Geometry check sheet. Reference: the model listing, model coordinates, mm. A direction names the side the tool comes from. Round coordinates to 2 decimals unless told otherwise and drop trailing zeros. Loops run counter-clockwise (first coordinate to the right, second up) from the corner with the lowest first, then second, coordinate; pieces in that order, holes last. Notation, with made-up numbers: M -25,86.25 L -9,86.25 A16 cw -9,98.25 Z; hole C 50.5,-26 d3. An arc over 180 degrees is marked long. Write item = value, one per line.
from build123d import *

# Parameters (mm, degrees)
SKETCH2_W            = 63.5
SKETCH2_H            = 63.5
BOSS_EXTRUDE1_DEPTH  = 2.54
BOSS_EXTRUDE2_DEPTH  = 2.54
SKETCH4_R            = 1.27
CUT_EXTRUDE1_DEPTH   = 2.54
BOSS_EXTRUDE3_DEPTH  = 2.54
BOSS_EXTRUDE4_DEPTH  = 2.54
EXTRUDE_THIN1_DEPTH  = 2.54
BOSS_EXTRUDE10_DEPTH = 2.54
SKETCH8_R            = 1.27
BOSS_EXTRUDE11_DEPTH = 42.418


with BuildPart() as part:
    # Sketch2 → Boss-Extrude1 (new body)
    with BuildSketch(Plane(origin=(0, 0, 0), x_dir=(1, 0, 0), z_dir=(0, 1, 0))):
        Rectangle(SKETCH2_W, SKETCH2_H)
    extrude(amount=BOSS_EXTRUDE1_DEPTH)

    # Sketch3 → Boss-Extrude2 (add)
    with BuildSketch(Plane(origin=(0, 17.145, 17.145), x_dir=(1, 0, 0), z_dir=(0, 0.707106781, 0.707106781))):
        Polygon((0, -20.654589078), (-12.7, -20.654589078), (-12.7, 42.845410922), (12.7, 42.845410922), (12.7, -20.654589078), align=None)
    extrude(amount=-BOSS_EXTRUDE2_DEPTH)

    # Sketch4 → Cut-Extrude1 (cut)
    with BuildSketch(Plane(origin=(0, 17.145, 17.145), x_dir=(1, 0, 0), z_dir=(0, 0.707106781, 0.707106781))):
        with Locations((0, 29.891410922)):
            Circle(SKETCH4_R)
        with Locations((-5.08, 29.891410922)):
            Circle(SKETCH4_R)
        with Locations((-10.16, 29.891410922)):
            Circle(SKETCH4_R)
        with Locations((-5.08, 23.287410922)):
            Circle(SKETCH4_R)
        with Locations((-5.08, 10.079410922)):
            Circle(SKETCH4_R)
        with Locations((0, 10.079410922)):
            Circle(SKETCH4_R)
        with Locations((5.08, 10.079410922)):
            Circle(SKETCH4_R)
        with Locations((10.16, 10.079410922)):
            Circle(SKETCH4_R)
        with Locations((5.08, -16.336589078)):
            Circle(SKETCH4_R)
        with Locations((-10.16, 36.495410922)):
            Circle(SKETCH4_R)
        with Locations((-5.08, 36.495410922)):
            Circle(SKETCH4_R)
        with Locations((0, 36.495410922)):
            Circle(SKETCH4_R)
        with Locations((5.08, 36.495410922)):
            Circle(SKETCH4_R)
        with Locations((10.16, 36.495410922)):
            Circle(SKETCH4_R)
        with Locations((10.16, 29.891410922)):
            Circle(SKETCH4_R)
        with Locations((5.08, 29.891410922)):
            Circle(SKETCH4_R)
        with Locations((-10.16, 23.287410922)):
            Circle(SKETCH4_R)
        with Locations((0, 23.287410922)):
            Circle(SKETCH4_R)
        with Locations((5.08, 23.287410922)):
            Circle(SKETCH4_R)
        with Locations((10.16, 23.287410922)):
            Circle(SKETCH4_R)
        with Locations((10.16, 16.683410922)):
            Circle(SKETCH4_R)
        with Locations((5.08, 16.683410922)):
            Circle(SKETCH4_R)
        with Locations((0, 16.683410922)):
            Circle(SKETCH4_R)
        with Locations((-5.08, 16.683410922)):
            Circle(SKETCH4_R)
        with Locations((-10.16, 16.683410922)):
            Circle(SKETCH4_R)
        with Locations((-10.16, 10.079410922)):
            Circle(SKETCH4_R)
        with Locations((10.16, 3.475410922)):
            Circle(SKETCH4_R)
        with Locations((5.08, 3.475410922)):
            Circle(SKETCH4_R)
        with Locations((0, 3.475410922)):
            Circle(SKETCH4_R)
        with Locations((-5.08, 3.475410922)):
            Circle(SKETCH4_R)
        with Locations((-10.16, 3.475410922)):
            Circle(SKETCH4_R)
        with Locations((-10.16, -3.128589078)):
            Circle(SKETCH4_R)
        with Locations((-5.08, -3.128589078)):
            Circle(SKETCH4_R)
        with Locations((0, -3.128589078)):
            Circle(SKETCH4_R)
        with Locations((5.08, -3.128589078)):
            Circle(SKETCH4_R)
        with Locations((10.16, -3.128589078)):
            Circle(SKETCH4_R)
        with Locations((10.16, -9.732589078)):
            Circle(SKETCH4_R)
        with Locations((5.08, -9.732589078)):
            Circle(SKETCH4_R)
        with Locations((0, -9.732589078)):
            Circle(SKETCH4_R)
        with Locations((-5.08, -9.732589078)):
            Circle(SKETCH4_R)
        with Locations((-10.16, -9.732589078)):
            Circle(SKETCH4_R)
        with Locations((-10.16, -16.336589078)):
            Circle(SKETCH4_R)
        with Locations((-5.08, -16.336589078)):
            Circle(SKETCH4_R)
        with Locations((0, -16.336589078)):
            Circle(SKETCH4_R)
        with Locations((10.16, -16.336589078)):
            Circle(SKETCH4_R)
    extrude(amount=-CUT_EXTRUDE1_DEPTH, mode=Mode.SUBTRACT)

    # Sketch5 → Boss-Extrude3 (add)
    with BuildSketch(Plane(origin=(0, 17.145, 17.145), x_dir=(1, 0, 0), z_dir=(0, 0.707106781, 0.707106781))):
        Polygon((12.7, 18.940681089), (12.7, 11.095410922), (27.502396542, 37.739724698), (24.17185732, 39.590024266), align=None)
        Polygon((27.500255446, -15.55009224), (12.7, 11.095410922), (12.7, 3.250490946), (24.17019797, -17.399774004), align=None)
    extrude(amount=-BOSS_EXTRUDE3_DEPTH)

    # Sketch6 → Boss-Extrude4 (add)
    with BuildSketch(Plane(origin=(0, 17.145, 17.145), x_dir=(1, 0, 0), z_dir=(0, 0.707106781, 0.707106781))):
        Polygon((-12.69936958, 18.940681064), (-12.7, 11.095410922), (-27.500255446, 37.740914083), (-24.169567551, 39.590946014), align=None)
        Polygon((-24.17185732, -17.399202422), (-12.7, 3.250140754), (-12.7, 11.095410922), (-27.502396542, -15.548902855), align=None)
    extrude(amount=-BOSS_EXTRUDE4_DEPTH)

    # Sketch7 → Extrude-Thin1 (add)
    with BuildSketch(Plane(origin=(0, 17.145, 17.145), x_dir=(1, 0, 0), z_dir=(0, 0.707106781, 0.707106781))):
        with BuildLine():
            ThreePointArc((-24.169567551, 39.590946014), (0.001261553, 45.709206507), (24.17185732, 39.590024266))
            Line((24.17185732, 39.590024266), (22.963279101, 37.355983378))
            ThreePointArc((22.963279101, 37.355983378), (0.001213122, 43.169206508), (-22.961074527, 37.356859039))
            Line((-22.961074527, 37.356859039), (-24.169567551, 39.590946014))
        make_face()
    extrude(amount=-EXTRUDE_THIN1_DEPTH)

    # Sketch7_6 → Boss-Extrude10 (add)
    with BuildSketch(Plane(origin=(0, 17.145, 17.145), x_dir=(1, 0, 0), z_dir=(0, 0.707106781, 0.707106781))):
        with BuildLine():
            Line((-24.17185732, -17.399202422), (-24.169567551, 39.590946014))
            ThreePointArc((-24.169567551, 39.590946014), (-41.917382675, 11.096584828), (-24.17185732, -17.399202422))
        make_face()
        with BuildLine():
            ThreePointArc((24.17185732, 39.590024266), (41.917233568, 11.095585974), (24.17185732, -17.398852317))
            Line((24.17185732, -17.398852317), (24.17185732, 39.590024266))
        make_face()
    extrude(amount=-BOSS_EXTRUDE10_DEPTH)

    # Sketch8 → Boss-Extrude11 (add)
    with BuildSketch(Plane(origin=(0, 2.54, 0), x_dir=(1, 0, 0), z_dir=(0, 1, 0))):
        with Locations((0, 12.7)):
            Circle(SKETCH8_R)
    extrude(amount=BOSS_EXTRUDE11_DEPTH)


solid = part.part
(1) Tool access check on faces 3 (the flat face through (0, 1, -31.75)), 4 (the flat face through (-18.516, 11.155, 21.364)), 5 (the flat face through (-0.078, 46.556, -14.037)), 6 (the flat face through (27.225, 5.156, 27.363)). Record the directions out of +Z, -Z, +X, -X, +Y, -Y that give a thin tool (end or side, any length) a straight path to the whole face; none if there is none.
Result set:
face_3 = -Z, +X, -X, +Y, -Y
face_4 = +Z
face_5 = none
face_6 = +Z, +X
(2) Release check for a two-part mould opening along Y. For faces 1 (the flat face through (31.75, 1, 0)), 2 (the cylindrical face through (-3.91, 37.05, -4.53)) record: released by +Y, released by -Y, zero draft, split by the parting line, or undercut.
Result set:
face_1 = zero draft
face_2 = undercut
(3) Sectioned sample at C-C on x = 0. State how many separate pieces and enclosed holes the cut face has, then the cut area to 3 significant figures.
Result set:
separate_pieces = 10
enclosed_holes = 0
area = 372 mm2
(4) Sectioned sample at B-B on x = -28.5. Record the cut outline in (y, z), then the cut area to 3 significant figures.
Result set:
outline = M 0,-31.75 L 2.54,-31.75 L 2.54,31.75 L 0,31.75 Z; M 4.86,25.83 L 41.52,-10.83 L 43.32,-9.03 L 6.66,27.63 Z
area = 293 mm2
(5) Depth check by flat-ended pin: pin 1 Ø8 at (x, y) = (14, 16) entering from +Z; pin 2 Ø8 at (x, y) = (-26, 13) entering from +Z; pin 3 Ø4 at (x, y) = (-31, 34.5) entering from -Z. Enter the tip coordinate at first touch or a pass-through.
Result set:
pin_1 = 22.07
pin_2 = 25.29
pin_3 = -5.8
(6) Sectioned sample at A-A on x = 19. Record the cut outline in (y, z).
Result set:
outline = M 0,-31.75 L 2.54,-31.75 L 2.54,31.75 L 0,31.75 Z; M 9.63,21.07 L 15.17,15.52 L 16.97,17.32 L 11.42,22.87 Z; M 31.21,-0.52 L 36.76,-6.06 L 38.56,-4.27 L 33.01,1.28 Z; M 43.12,-12.42 L 45.06,-14.37 L 46.86,-12.57 L 44.91,-10.62 Z
(7) Material ranges on line 1 along X through (y, z) = (35, -1.5); line 2 along Y through (x, z) = (30, 27.5); line 3 along X through (y, z) = (2, 12), recorded low to high. Write a range as from..to.
Result set:
line_1 = -38.3..-24.17, -20.87..-16.51, -12.7..12.7, 16.52..20.87, 24.17..38.3
line_2 = 0..2.54
line_3 = -31.75..31.75
